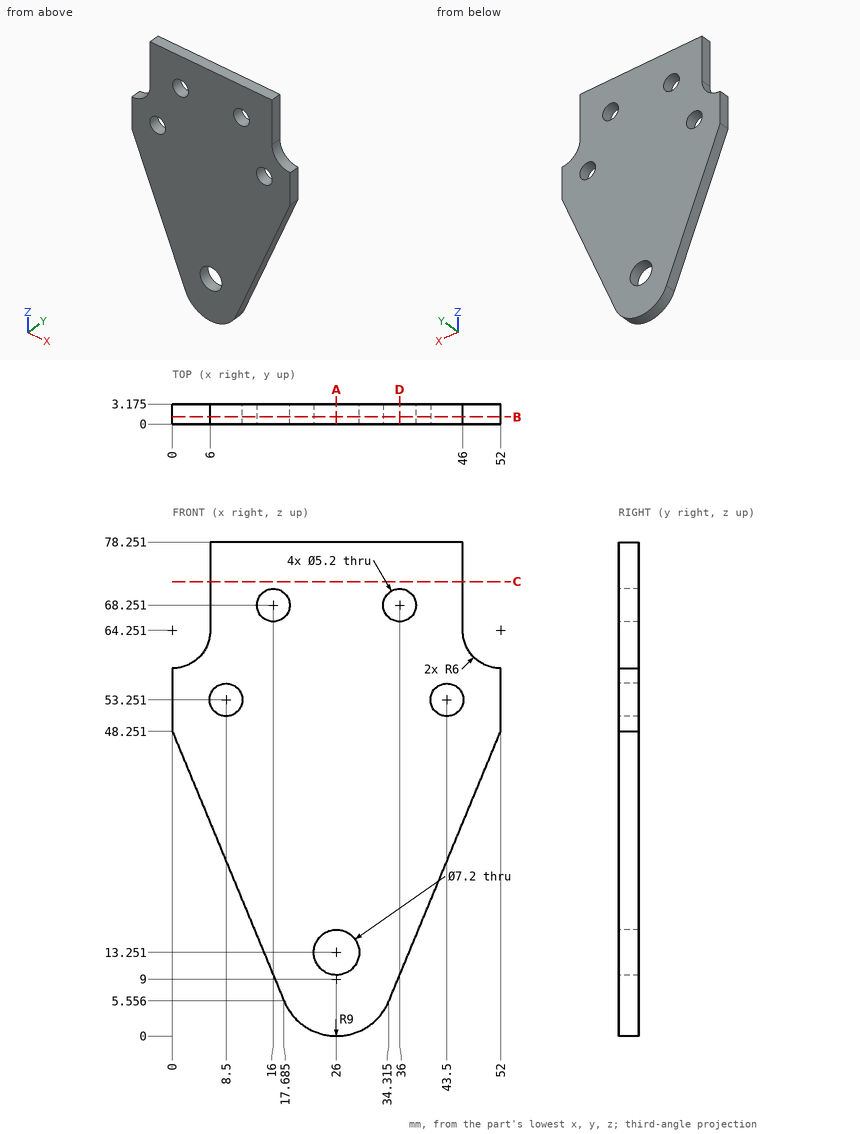
The drawing under review shows one solid part. Ordinate dimensions are in mm from its lowest x, y, z. Coordinates: 2 decimals unless noted, no trailing zeros. Loops run counter-clockwise (first coordinate to the right, second up) from the corner with the lowest first, then second, coordinate; pieces in that order, holes last. Notation, with made-up numbers: (60, 8) -> (109, 8) arc R30 cw to (109, 42) -> close; hole circle Ø3 at (44, 13.25). An arc over 180 degrees is marked (long way). Answer as a JSON object with one key per item and string values.
Q1. To check wall thickness, follow L1, parallel to Z at x = 26, y = 2.2; L2, parallel to X at y = 0.9, z = 53; L3, parallel to X at y = 3.05, z = 55.5 (1 decimal). State the ranges of each line that lie inside material, in increasing order.
Answer block:
{"L1": "z = 0 to 9.65, 16.85 to 78.25", "L2": "x = 0 to 5.91, 11.09 to 40.91, 46.09 to 52", "L3": "x = 0 to 7.2, 9.8 to 42.2, 44.8 to 52"}
Q2. Clearance check with flat-ended pins moving along their axes: pin 1 Ø1 at (y, z) = (1, 70) entering from -X; pin 2 Ø1.6 at (y, z) = (1, 73.5) entering from +X; pin 3 Ø1.5 at (y, z) = (2, 63.5) entering from +X. State where each tip first meets the part, or that it passes through.
Answer block:
{"pin 1": "stops at x = 6", "pin 2": "stops at x = 46", "pin 3": "stops at x = 46.19"}
Q3. Take a section at B-B on y = 1.15. Give the boundary of the cut face in (x, z) (1 decimal).
Answer block:
{"outline": "(0, 48.3) -> (17.7, 5.6) arc R9 ccw to (34.3, 5.6) -> (52, 48.3) -> (52, 58.3) arc R6 cw to (46, 64.3) -> (46, 78.3) -> (6, 78.3) -> (6, 64.3) arc R6 cw to (0, 58.3) -> close; hole circle Ø5.2 at (8.5, 53.3); hole circle Ø5.2 at (16, 68.3); hole circle Ø7.2 at (26, 13.3); hole circle Ø5.2 at (36, 68.3); hole circle Ø5.2 at (43.5, 53.3)"}
Q4. Take a section at A-A on x = 26. Give the boundary of the cut face in (y, z) (1 decimal).
Answer block:
{"outline": "(0, 0) -> (3.2, 0) -> (3.2, 9.7) -> (0, 9.7) -> close; (0, 16.9) -> (3.2, 16.9) -> (3.2, 78.3) -> (0, 78.3) -> close"}
Q5. Take a section at D-D on x = 36. Give the boundary of the cut face in (y, z) (1 decimal).
Answer block:
{"outline": "(0, 9.6) -> (3.2, 9.6) -> (3.2, 65.7) -> (0, 65.7) -> close; (0, 70.9) -> (3.2, 70.9) -> (3.2, 78.3) -> (0, 78.3) -> close"}
Q6. Take a section at C-C on z = 72. Give the boundary of the cut face in (x, y) (1 decimal).
Answer block:
{"outline": "(6, 0) -> (46, 0) -> (46, 3.2) -> (6, 3.2) -> close"}
